Build history of the part. All positions in model axes, mm. A direction names the side the tool comes from. Coordinates: 2 decimals unless noted, no trailing zeros. Loops run counter-clockwise (first coordinate to the right, second up) from the corner with the lowest first, then second, coordinate; pieces in that order, holes last.
(1) Wall check: L1, parallel to X at y = 10, z = 1.8; L2, parallel to Z at x = 1.75, y = 35; L3, parallel to Y at x = 2.5, z = 0.3. Give the ranges that are in metal, low to high.
(2) Slice it at B-B (y = 15). Give the cut face in (x, z), and give its area (3 significant figures).
(3) Tool access for faces 1 (the face through (0, 16, 2)), 2 (the face through (2, 18, 1)): list every direction of +Z, -Z, +X, -X, +Y, -Y with a clear straight run to the whole face (end or side of a thin tool).
(4) Flat gauge pin, fed straight in: P1, Ø1, axis at y = 20, z = 1, coming from the -X side. Where does the tip first touch, or does it go through?
(5) Two-plate mould, pull along Y, no slides. Class faces 3 (the face through (-1.5, 0.07, 0.99)), 4 (the face through (-1.2, 37, 0.8)), 5 (the face through (-2, 19, 1)): pulls with the +Y half, pulls with the -Y half, needs draft (parallel to the pull), parting line crosses it, or undercut.
(6) Slice it at A-A (y = 0). Give the cut face in (x, z).
(7) Slice it at C-C (x = 2.5). Give the cut face in (y, z).
from build123d import *

# Parameters (mm, degrees)
SKETCH_R     = 1.5
PAD_DEPTH    = 2
POCKET_DEPTH = 2.5
FILLET_R     = 0.5


with BuildPart() as part:
    # Sketch → Pad (new body)
    with BuildSketch(Plane.XY):
        with BuildLine():
            ThreePointArc((-2, 2.236068), (0, -3), (2, 2.236068))
            Line((2, 2.236068), (2, 35))
            Line((0, 40), (2, 35))
            Line((0, 40), (-2, 35))
            Line((-2, 35), (-2, 2.236068))
        make_face()
        Circle(SKETCH_R, mode=Mode.SUBTRACT)
    extrude(amount=PAD_DEPTH)

    # Sketch001 → Pocket (cut, symmetric)
    with BuildSketch(Plane.YZ):
        Polygon((40.364792, 0), (32.17564, 3.019657), (42.446777, 4.153183), align=None)
    extrude(amount=POCKET_DEPTH, both=True, mode=Mode.SUBTRACT)

    # Fillet
    fillet_edges = [part.edges().sort_by_distance(p)[0] for p in [
        (-1.5, 0, 2),
        (-1.5, 0, 0),
    ]]
    fillet(fillet_edges, radius=FILLET_R)


solid = part.part
Response values:
1. L1: x = -2 to 2
1. L2: z = 0 to 1.98
1. L3: y = -1.66 to 1.66
2. outline: (-2, 0) - (2, 0) - (2, 2) - (-2, 2) - close
2. area: 8.00 mm2
3. face 1: +Z, +X, -X, +Y, -Y
3. face 2: +Z, -Z, +X, +Y
4. P1: stops at x = -2
5. face 3: undercut
5. face 4: pulls with the +Y half
5. face 5: needs draft
6. outline: (-3, 0) - (-2, 0) arc R0.5 ccw to (-1.5, 0.5) - (-1.5, 1.5) arc R0.5 ccw to (-2, 2) - (-3, 2) - close; (1.5, 0.5) arc R0.5 ccw to (2, 0) - (3, 0) - (3, 2) - (2, 2) arc R0.5 ccw to (1.5, 1.5) - close
7. outline: (-1.66, 0) - (1.66, 0) - (1.66, 2) - (-1.66, 2) - close
